```python
from build123d import *

# Parameters (mm, degrees)
F1_DEPTH = 5.08
F2_R     = 3.175
F3_DEPTH = 25.4
F4_R     = 12.7
F5_R     = 1.27
F6_R     = 0.624085
F6_R_2   = 0.644675
F6_R_3   = 0.690693
F6_R_4   = 0.661099
F6_R_5   = 0.595245
F6_R_6   = 0.666861
F6_R_7   = 0.612219
F6_R_8   = 0.570033
F6_R_9   = 0.614095
F6_R_10  = 0.689377
F6_R_11  = 0.615925
F6_R_12  = 0.655138
F6_R_13  = 0.735757
F6_R_14  = 0.585279
F7_DEPTH = 6.35


with BuildPart() as f1:
    # F0 (on Front) → F1 (new body)
    with BuildSketch(Plane.XZ):
        with BuildLine():
            Line((19.05, -25.4), (19.05, 25.4))
            Line((19.05, 25.4), (-19.05, 25.4))
            Line((-19.05, 25.4), (-19.05, -14.215613))
            ThreePointArc((-19.05, -14.215613), (-5.783979, -22.294952), (9.435144, -25.4))
            Line((9.435144, -25.4), (19.05, -25.4))
        make_face()
    extrude(amount=F1_DEPTH)

    # F2 (on face) → F3 (cut)
    with BuildSketch(Plane.XZ.offset(5.08)):
        Circle(F2_R)
    extrude(amount=-F3_DEPTH, mode=Mode.SUBTRACT)

    # F4
    f4_edges = [f1.edges().sort_by_distance(p)[0] for p in [
        (19.05, -2.54, 25.4),
        (-19.05, -2.54, 25.4),
    ]]
    fillet(f4_edges, radius=F4_R)

    # F5
    f5_edges = [f1.edges().sort_by_distance(p)[0] for p in [
        (19.05, -2.54, -25.4),
    ]]
    fillet(f5_edges, radius=F5_R)

    # F6 (on face) → F7 (join)
    with BuildSketch(Plane.XZ.offset(5.08)):
        with Locations((-16.64902, -16.17935)):
            Circle(F6_R)
        with Locations((-14.501234, -17.718923)):
            Circle(F6_R_2)
        with Locations((-11.7464, -19.433464)):
            Circle(F6_R_3)
        with Locations((-9.440057, -20.668933)):
            Circle(F6_R_4)
        with Locations((-7.113972, -21.748141)):
            Circle(F6_R_5)
        with Locations((-4.741597, -22.689453)):
            Circle(F6_R_6)
        with Locations((-2.305846, -23.499407)):
            Circle(F6_R_7)
        with Locations((0, -24.127949)):
            Circle(F6_R_8)
        with Locations((2.657019, -24.693049)):
            Circle(F6_R_9)
        with Locations((5.553329, -25.122012)):
            Circle(F6_R_10)
        with Locations((7.93359, -25.332349)):
            Circle(F6_R_11)
        with Locations((10.451948, -25.4)):
            Circle(F6_R_12)
        with Locations((13.607572, -25.4)):
            Circle(F6_R_13)
        with Locations((16.427536, -25.4)):
            Circle(F6_R_14)
    extrude(amount=-F7_DEPTH)


solid = f1.part
```
Input: part model. Units: mm. Frame: model coordinates. A direction names the side the tool comes from. Round coordinates to 2 decimals unless told otherwise and drop trailing zeros. Loops run counter-clockwise (first coordinate to the right, second up) from the corner with the lowest first, then second, coordinate; pieces in that order, holes last.
1) Pull-direction query (X, two-part tool) for faces 1 (the cylindrical face through (18.688, -2.576, -25.018)), 2 (the flat face through (15, -3, -25.4)), 3 (the flat face through (3, 1.27, -25)), 4 (the cylindrical face through (4.053, -2.504, -24.924)); classes: released by +X, released by -X, zero draft, split by the parting line, or undercut.
Ans:
face 1: released by +X
face 2: undercut
face 3: zero draft
face 4: undercut
2) Section query A-A on z = 0. Return the cut outline in (x, y) (3 decimals), plus the area to 3 significant figures.
Ans:
outline: (-19.05, -5.08) - (-3.175, -5.08) - (-3.175, 0) - (-19.05, 0) - close; (3.175, -5.08) - (19.05, -5.08) - (19.05, 0) - (3.175, 0) - close
area: 161 mm2
3) Section query D-D on z = 13.5. Return the cut outline in (x, y).
Ans:
outline: (-19.02, -5.08) - (19.02, -5.08) - (19.02, 0) - (-19.02, 0) - close
4) Section query B-B on x = 0. Return the cut outline in (y, z) (3 decimals), plus the area to 3 significant figures.
Ans:
outline: (-5.08, -24.698) - (1.27, -24.698) - (1.27, -23.558) - (0, -23.558) - (0, -3.175) - (-5.08, -3.175) - close; (-5.08, 3.175) - (0, 3.175) - (0, 25.4) - (-5.08, 25.4) - close
area: 224 mm2
5) Section query C-C on x = 13.5. Return the cut outline in (y, z), plus the area to 3 significant figures.
Ans:
outline: (-5.08, -26.13) - (1.27, -26.13) - (1.27, -24.67) - (0, -24.67) - (0, 23.2) - (-5.08, 23.2) - close
area: 252 mm2
6) Material intervals for line 1 (Z direction, x = 0, y = -1.6) (3 decimals); line 2 (Y direction, x = -9, z = -19); line 3 (X direction, y = -0.5, z = 1), sorted ascending.
Ans:
line 1: z = -24.698 to -3.175, 3.175 to 25.4
line 2: y = -5.08 to 0
line 3: x = -19.05 to -3.01, 3.01 to 19.05
7) Set-up query: faces 5 (the cylindrical face through (2.52, -1.24, -25.29)), 6 (the flat face through (0, -3, 25.4)), 7 (the flat face through (12, -3, -25.4)). Return all of +Z, -Z, +X, -X, +Y, -Y with unobstructed straight access to the full face (end or side cutting, diameter ignored); none if empty.
Ans:
face 5: +Y
face 6: +Z, +X, -X, +Y, -Y
face 7: -Z, +Y, -Y
8) Pin query (flat end, axial travel): pin 1 (0.6 mm diameter, centred on x = 17.5, y = -3, fed in from -Z); pin 2 (10 mm diameter, centred on x = 0, z = 0, fed in from -Y); pin 3 (2 mm diameter, centred on x = 0.5, y = -1, fed in from -Z). Return the tip coordinate at first contact, or that it passes through.
Ans:
pin 1: stops at z = -25.4
pin 2: stops at y = -5.08
pin 3: stops at z = -24.7
